from build123d import *

# Parameters (mm, degrees)
F1_DEPTH = 2.54


with BuildPart() as f1:
    # F0 (on Top) → F1 (new body)
    with BuildSketch(Plane.XY):
        with BuildLine():
            ThreePointArc((0, 48.26), (34.124973, 34.124973), (48.26, 0))
            Line((48.26, 0), (150.8125, 0))
            ThreePointArc((150.8125, 0), (106.183757, 106.183757), (0, 150.8125))
            Line((0, 150.8125), (0, 48.26))
        make_face()
        with BuildLine():
            Line((55.245, 127.75815), (55.245, 13.362749))
            ThreePointArc((55.245, 13.362749), (51.503135, 24.041635), (45.72, 33.767657))
            Line((45.72, 33.767657), (45.72, 131.559986))
            ThreePointArc((45.72, 131.559986), (50.517399, 129.746504), (55.245, 127.75815))
        make_face(mode=Mode.SUBTRACT)
        with BuildLine():
            Line((74.93, 6.35), (65.405, 6.35))
            Line((65.405, 6.35), (65.405, 122.762105))
            ThreePointArc((65.405, 122.762105), (70.223809, 120.019687), (74.93, 117.088215))
            Line((74.93, 117.088215), (74.93, 6.35))
        make_face(mode=Mode.SUBTRACT)
        with BuildLine():
            ThreePointArc((124.46, 60.893818), (129.865191, 48.162763), (133.985, 34.959619))
            Line((133.985, 34.959619), (133.985, 6.867618))
            ThreePointArc((133.985, 6.867618), (132.755827, 6.480751), (131.47386, 6.35))
            Line((131.47386, 6.35), (124.46, 6.35))
            Line((124.46, 6.35), (124.46, 60.893818))
        make_face(mode=Mode.SUBTRACT)
        with BuildLine():
            Line((104.775, 6.35), (104.775, 90.942553))
            ThreePointArc((104.775, 90.942553), (109.712471, 84.84681), (114.3, 78.483534))
            Line((114.3, 78.483534), (114.3, 6.35))
            Line((114.3, 6.35), (104.775, 6.35))
        make_face(mode=Mode.SUBTRACT)
        with BuildLine():
            Line((94.615, 6.35), (85.09, 6.35))
            Line((85.09, 6.35), (85.09, 109.809109))
            ThreePointArc((85.09, 109.809109), (89.944941, 105.810796), (94.615, 101.598016))
            Line((94.615, 101.598016), (94.615, 6.35))
        make_face(mode=Mode.SUBTRACT)
        with BuildLine():
            ThreePointArc((35.56, 44.340269), (30.952351, 47.671009), (26.035, 50.524765))
            Line((26.035, 50.524765), (26.035, 137.005573))
            ThreePointArc((26.035, 137.005573), (30.81719, 135.965077), (35.56, 134.757713))
            Line((35.56, 134.757713), (35.56, 44.340269))
        make_face(mode=Mode.SUBTRACT)
        with BuildLine():
            ThreePointArc((11.423732, 55.678285), (7.779289, 57.885092), (6.35, 61.898706))
            Line((6.35, 61.898706), (6.35, 132.616219))
            ThreePointArc((6.35, 132.616219), (8.451575, 137.335688), (13.365238, 138.931277))
            ThreePointArc((13.365238, 138.931277), (14.620769, 138.793276), (15.875, 138.643929))
            Line((15.875, 138.643929), (15.875, 54.576162))
            ThreePointArc((15.875, 54.576162), (13.660485, 55.172133), (11.423732, 55.678285))
        make_face(mode=Mode.SUBTRACT)
    extrude(amount=F1_DEPTH)


solid = f1.part
Geometry: final body of the model. Coordinates: model frame, mm. A direction names the side the tool comes from. Round coordinates to 2 decimals unless told otherwise and drop trailing zeros. Loops run counter-clockwise (first coordinate to the right, second up) from the corner with the lowest first, then second, coordinate; pieces in that order, holes last.
Q1. Pin query (flat end, axial travel): P1, Ø1, axis at x = 104.5, y = 57, coming from the -Z side; P2, Ø4, axis at x = 77.5, y = 133, coming from the -Z side; P3, Ø1.3, axis at y = 76, z = 2, coming from the +X side; P4, Ø0.8, axis at x = 70.5, z = 2, coming from the +Y side. Return the tip coordinate at first contact, or that it passes through.
Q2. Access query for faces 1 (the cylindrical face through (8.4, 137.29, 1.25)), 2 (the cylindrical face through (107.347, 105.008, 1.252)). Directions: +Z, -Z, +X, -X, +Y, -Y. A direction counts if a zero-diameter tool reaches every point of the face in a straight line with its end or side. Return the directions, or none.
Q3. Section B-B on y = 52.5. Return loops of the section in (x, z) (3 decimals), plus the area to 3 significant figures.
Q4. Section A-A on x = 89. Return loops of the section in (y, z), plus the area to 3 significant figures.
Q5. Material intervals for L1, parallel to X at y = 13, z = 2.2 (3 decimals); L2, parallel to X at y = 101, z = 0.5 (3 decimals); L3, parallel to X at y = 118, z = 1.05 (3 decimals), sorted ascending.
Q6. Section D-D on x = 70. Return loops of the section in (y, z).
Q7. Pull-direction query (Y, two-part tool) for faces 3 (the cylindrical face through (33.748, 34.498, 1.252)), 4 (the cylindrical face through (7.818, 57.838, 1.252)), 5 (the flat face through (58, 76, 2.54)); classes: released by +Y, released by -Y, zero draft, split by the parting line, or undercut.
Q8. Section C-C on z = 0.75. State how many separate pieces and enclosed holes the cut face has, plus the area to 3 significant figures.
Evaluation:
1. P1: stops at z = 0
1. P2: passes through
1. P3: stops at x = 129.98
1. P4: stops at y = 132.91
2. face 1: +Z, -Z
2. face 2: +Z, -Z, +X, +Y
3. outline: (0, 0) - (26.035, 0) - (26.035, 2.54) - (0, 2.54) - close; (35.56, 0) - (45.72, 0) - (45.72, 2.54) - (35.56, 2.54) - close; (55.245, 0) - (65.405, 0) - (65.405, 2.54) - (55.245, 2.54) - close; (74.93, 0) - (85.09, 0) - (85.09, 2.54) - (74.93, 2.54) - close; (94.615, 0) - (104.775, 0) - (104.775, 2.54) - (94.615, 2.54) - close; (114.3, 0) - (124.46, 0) - (124.46, 2.54) - (114.3, 2.54) - close; (128.19, 0) - (140.903, 0) - (140.903, 2.54) - (128.19, 2.54) - close
3. area: 227 mm2
4. outline: (0, 0) - (6.35, 0) - (6.35, 2.54) - (0, 2.54) - close; (106.62, 0) - (120.98, 0) - (120.98, 2.54) - (106.62, 2.54) - close
4. area: 52.6 mm2
5. L1: x = 46.476 to 65.405, 74.93 to 85.09, 94.615 to 104.775, 114.3 to 124.46, 133.985 to 150.122
5. L2: x = 0 to 6.35, 15.875 to 26.035, 35.56 to 45.72, 55.245 to 65.405, 74.93 to 85.09, 94.615 to 111.129
5. L3: x = 0 to 6.35, 15.875 to 26.035, 35.56 to 45.72, 55.245 to 65.405, 73.51 to 92.901
6. outline: (0, 0) - (6.35, 0) - (6.35, 2.54) - (0, 2.54) - close; (120.15, 0) - (132.96, 0) - (132.96, 2.54) - (120.15, 2.54) - close
7. face 3: released by -Y
7. face 4: undercut
7. face 5: zero draft
8. separate pieces: 1
8. enclosed holes: 7
8. area: 10,100 mm2
